```python
from build123d import *

# Parameters (mm, degrees)
SERVO_SHELF_START                        = -27.480025
SKETCH1_W                                = 48
SKETCH1_H                                = 38
SKETCH1_W_2                              = 13
SKETCH1_H_2                              = 24.35
SERVO_SHELF_DEPTH                        = 3
OUTBOARD_RISER_START                     = -25.480025
SKETCH2_W                                = 6
SKETCH2_H                                = 14
OUTBOARD_RISER_DEPTH                     = 24.480025
PLATE_ATTACHMENT_FOOT_START              = -2
SKETCH3_W                                = 20
SKETCH3_H                                = 14
PLATE_ATTACHMENT_FOOT_DEPTH              = 2
SKETCH4_R                                = 1.45
SERVO_PAD_D2P9_DEPTH                     = 2.01
SKETCH5_R                                = 2.6
SERVO_PAD_CSK_D5P2_90DEG_DEPTH           = 1.15
SERVO_PAD_CSK_D5P2_90DEG_DRAFT           = -45
SERVO_PAD_CSK_D5P2_90DEG_PROFILE_2_DEPTH = 1.15
SERVO_PAD_CSK_D5P2_90DEG_PROFILE_2_DRAFT = -45
SERVO_EAR_SUPPORTS_H2P2_START            = -24.480025
SKETCH6_R                                = 2.5
SERVO_EAR_SUPPORTS_H2P2_DEPTH            = 2.2
SKETCH7_R                                = 1.2
SERVO_EAR_D2P4_THROUGH_DEPTH             = 5.21


with BuildPart() as part:
    # Sketch1 → Servo_Shelf (new body)
    with BuildSketch(Plane.XY.offset(SERVO_SHELF_START)):
        with Locations((-46, 19)):
            Rectangle(SKETCH1_W, SKETCH1_H)
        with Locations((-60, 18.825)):
            Rectangle(SKETCH1_W_2, SKETCH1_H_2, mode=Mode.SUBTRACT)
    extrude(amount=SERVO_SHELF_DEPTH)

    # Sketch2 → Outboard_Riser (add)
    with BuildSketch(Plane.XY.offset(OUTBOARD_RISER_START)):
        with Locations((-37, 21)):
            Rectangle(SKETCH2_W, SKETCH2_H)
    extrude(amount=OUTBOARD_RISER_DEPTH)

    # Sketch3 → Plate_Attachment_Foot (add)
    with BuildSketch(Plane.XY.offset(PLATE_ATTACHMENT_FOOT_START)):
        with Locations((-30, 21)):
            Rectangle(SKETCH3_W, SKETCH3_H)
    extrude(amount=PLATE_ATTACHMENT_FOOT_DEPTH)

    # Sketch4 → Servo_Pad_D2p9 (cut)
    with BuildSketch(Plane(origin=(0, 0, -2), x_dir=(-1, 0, 0), z_dir=(0, 0, -1))):
        with Locations((25, 18)):
            Circle(SKETCH4_R)
        with Locations((25, 25)):
            Circle(SKETCH4_R)
    extrude(amount=-SERVO_PAD_D2P9_DEPTH, mode=Mode.SUBTRACT)


with BuildPart() as servo_pad_csk_d5p2_90deg_tool:
    # Sketch5 → Servo_Pad_CSK_D5p2_90deg (with draft: the straight prism first)
    with BuildSketch(Plane(origin=(0, 0, -2), x_dir=(-1, 0, 0), z_dir=(0, 0, -1))):
        with Locations((25, 18)):
            Circle(SKETCH5_R)
    extrude(amount=-SERVO_PAD_CSK_D5P2_90DEG_DEPTH)
    # Servo_Pad_CSK_D5p2_90deg: the draft: its side faces are tilted about the plane it starts from
    servo_pad_csk_d5p2_90deg_sides = [servo_pad_csk_d5p2_90deg_tool.faces().sort_by_distance(p)[0] for p in [
        (-22.4, 18, -1.425),
    ]]
    draft(servo_pad_csk_d5p2_90deg_sides, Plane(origin=(0, 0, -2), x_dir=(-1, 0, 0), z_dir=(0, 0, -1)), SERVO_PAD_CSK_D5P2_90DEG_DRAFT)


with BuildPart() as part_1:
    add(part.part)

    # Servo_Pad_CSK_D5p2_90deg: cut by servo_pad_csk_d5p2_90deg_tool
    add(servo_pad_csk_d5p2_90deg_tool.part, mode=Mode.SUBTRACT)


with BuildPart() as servo_pad_csk_d5p2_90deg_profile_2_tool:
    # Sketch5 → Servo_Pad_CSK_D5p2_90deg profile 2 (with draft: the straight prism first)
    with BuildSketch(Plane(origin=(0, 0, -2), x_dir=(-1, 0, 0), z_dir=(0, 0, -1))):
        with Locations((25, 25)):
            Circle(SKETCH5_R)
    extrude(amount=-SERVO_PAD_CSK_D5P2_90DEG_PROFILE_2_DEPTH)
    # Servo_Pad_CSK_D5p2_90deg profile 2: the draft: its side faces are tilted about the plane it starts from
    servo_pad_csk_d5p2_90deg_profile_2_sides = [servo_pad_csk_d5p2_90deg_profile_2_tool.faces().sort_by_distance(p)[0] for p in [
        (-22.4, 25, -1.425),
    ]]
    draft(servo_pad_csk_d5p2_90deg_profile_2_sides, Plane(origin=(0, 0, -2), x_dir=(-1, 0, 0), z_dir=(0, 0, -1)), SERVO_PAD_CSK_D5P2_90DEG_PROFILE_2_DRAFT)


with BuildPart() as part_2:
    add(part_1.part)

    # Servo_Pad_CSK_D5p2_90deg profile 2: cut by servo_pad_csk_d5p2_90deg_profile_2_tool
    add(servo_pad_csk_d5p2_90deg_profile_2_tool.part, mode=Mode.SUBTRACT)

    # Sketch6 → Servo_Ear_Supports_H2p2 (add)
    with BuildSketch(Plane.XY.offset(SERVO_EAR_SUPPORTS_H2P2_START)):
        with Locations(Location((-60, 4.55, 0), (0, 0, 122.859880379))):
            Circle(SKETCH6_R)
        with Locations(Location((-60, 32.75, 0), (0, 0, 224.427004001))):
            Circle(SKETCH6_R)
    extrude(amount=SERVO_EAR_SUPPORTS_H2P2_DEPTH)

    # Sketch7 → Servo_Ear_D2p4_Through (cut)
    with BuildSketch(Plane.XY.offset(-22.280025)):
        with Locations((-60, 4.55)):
            Circle(SKETCH7_R)
        with Locations((-60, 32.75)):
            Circle(SKETCH7_R)
    extrude(amount=-SERVO_EAR_D2P4_THROUGH_DEPTH, mode=Mode.SUBTRACT)


solid = part_2.part
```
Verification items for the finished model (mm, model axes). A direction names the side the tool comes from. Give positions to 0.01 mm unless a question says otherwise; leave off trailing zeros. Order: outer loops, then holes, each group sorted by start corner. A loop starts at its lowest first (then second) coordinate and runs counter-clockwise, first axis right, second up. Notation, with made-up numbers: (43.25, 87) -> (49.25, 87) arc R8 ccw to (49.25, 98) -> close; hole circle Ø9 at (-37.5, -38). An arc over 180 degrees is marked (long way). Use a Markdown table: item, result.
1) Tool access check on faces 4 (the flat face through (-40, 21, -12)), 5 (the flat face through (-35, 28, -10)), 6 (the flat face through (-35, 14, -10)). Record the directions out of +Z, -Z, +X, -X, +Y, -Y that give a thin tool (end or side, any length) a straight path to the whole face; none if there is none.
Results:
| item | result |
|---|---|
| face 4 | +Z, -X, +Y, -Y |
| face 5 | +Z, +X, -X, +Y |
| face 6 | +Z, +X, -X, -Y |
2) Mould release check, pull along Z, two halves, no side actions. Record for faces 1 (the flat face through (-30, 21, 0)), 2 (the flat face through (-27, 21, -2)), 3 (the flat face through (-46, 0, -26)): pulls with the +Z half, pulls with the -Z half, needs draft (parallel to the pull), parting line crosses it, or undercut.
Results:
| item | result |
|---|---|
| face 1 | pulls with the +Z half |
| face 2 | undercut |
| face 3 | needs draft |
3) Depth check by flat-ended pin: pin 1 Ø3.5 at (y, z) = (14, -26.5) entering from +X; pin 2 Ø2.5 at (x, y) = (-60.5, 32.5) entering from +Z; pin 3 Ø2 at (y, z) = (22.5, -17) entering from +X; pin 4 Ø1 at (x, y) = (-65, 28.5) entering from +Z. Enter the tip coordinate at first touch or a pass-through.
Results:
| item | result |
|---|---|
| pin 1 | x = -22 |
| pin 2 | z = -22.28 |
| pin 3 | x = -34 |
| pin 4 | through |
4) Section check B-B, the plane y = 4.55. Record the boundary of the cut face in (x, z), then the cut area to 3 significant figures.
Results:
| item | result |
|---|---|
| outline | (-70, -27.48) -> (-61.2, -27.48) -> (-61.2, -22.28) -> (-62.5, -22.28) -> (-62.5, -24.48) -> (-70, -24.48) -> close; (-58.8, -27.48) -> (-22, -27.48) -> (-22, -24.48) -> (-57.5, -24.48) -> (-57.5, -22.28) -> (-58.8, -22.28) -> close |
| area | 143 mm² |
5) Section check A-A, the plane x = -60. Record the boundary of the cut face in (y, z).
Results:
| item | result |
|---|---|
| outline | (0, -27.48) -> (3.35, -27.48) -> (3.35, -22.28) -> (2.05, -22.28) -> (2.05, -24.48) -> (0, -24.48) -> close; (5.75, -27.48) -> (6.65, -27.48) -> (6.65, -24.48) -> (7.05, -24.48) -> (7.05, -22.28) -> (5.75, -22.28) -> close; (30.25, -24.48) -> (31, -24.48) -> (31, -27.48) -> (31.55, -27.48) -> (31.55, -22.28) -> (30.25, -22.28) -> close; (33.95, -27.48) -> (38, -27.48) -> (38, -24.48) -> (35.25, -24.48) -> (35.25, -22.28) -> (33.95, -22.28) -> close |
6) Material ranges on probe 1 along Y at (x, z) = (-25, -0.7); probe 2 along Y at (x, z) = (-60, -24); probe 3 along Y at (x, z) = (-60, -25.8), recorded low to high.
Results:
| item | result |
|---|---|
| probe 1 | 14 to 16.55, 19.45 to 23.55, 26.45 to 28 |
| probe 2 | 2.05 to 3.35, 5.75 to 7.05, 30.25 to 31.55, 33.95 to 35.25 |
| probe 3 | 0 to 3.35, 5.75 to 6.65, 31 to 31.55, 33.95 to 38 |
7) Section check C-C, the plane y = 25. Record the boundary of the cut face in (x, z).
Results:
| item | result |
|---|---|
| outline | (-70, -27.48) -> (-66.5, -27.48) -> (-66.5, -24.48) -> (-70, -24.48) -> close; (-53.5, -27.48) -> (-22, -27.48) -> (-22, -24.48) -> (-34, -24.48) -> (-34, -2) -> (-27.6, -2) -> (-26.45, -0.85) -> (-26.45, 0) -> (-40, 0) -> (-40, -24.48) -> (-53.5, -24.48) -> close; (-23.55, -0.85) -> (-22.4, -2) -> (-20, -2) -> (-20, 0) -> (-23.55, 0) -> close |
8) Section check D-D, the plane x = -25. Record the boundary of the cut face in (y, z), then the cut area to 3 significant figures.
Results:
| item | result |
|---|---|
| outline | (0, -27.48) -> (38, -27.48) -> (38, -24.48) -> (0, -24.48) -> close; (14, -2) -> (15.4, -2) -> (16.55, -0.85) -> (16.55, 0) -> (14, 0) -> close; (19.45, -0.85) -> (20.6, -2) -> (22.4, -2) -> (23.55, -0.85) -> (23.55, 0) -> (19.45, 0) -> close; (26.45, -0.85) -> (27.6, -2) -> (28, -2) -> (28, 0) -> (26.45, 0) -> close |
| area | 128 mm² |
